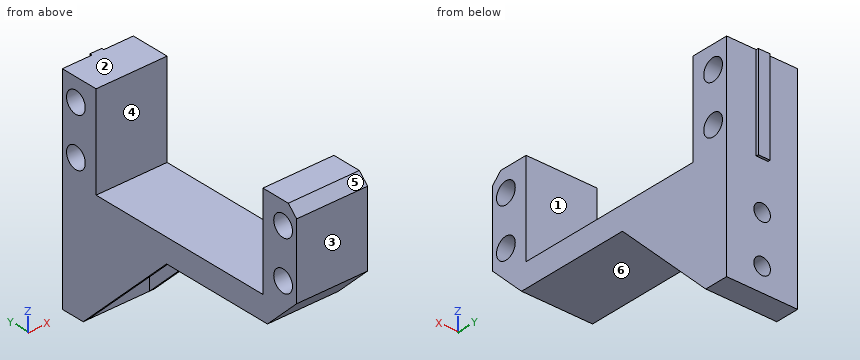
```python
from build123d import *

# Parameters (mm, degrees)
SKETCH019_R             = 2.25
PAD011_DEPTH            = 15
SKETCH020_W             = 20
SKETCH020_H             = 13
POCKET005_DEPTH         = 20
CHAMFER_SIZE            = 19.99
SKETCH021_R             = 1.75
POCKET006_DEPTH         = 5
SKETCH022_W             = 19.8
SKETCH022_H             = 2.5
PAD012_DEPTH            = 0.5
CHAMFER001_SIZE         = 7
CHAMFER002_SIZE         = 2
BODY003_PLACEMENT_ANGLE = 180


with BuildPart() as part:
    # Sketch019 → Pad011 (new body)
    with BuildSketch(Plane.YZ):
        Polygon((-20.02, -9.9), (-28.12, -9.9), (-28.12, 14.9), (3.12, 14.9), (3.12, 34.9), (23.12, 34.9), (28.12, 34.9), (28.12, -9.9), (20.02, -9.9), (20.02, 9.9), (-20.02, 9.9), align=None)
        with Locations((-24.87, -5.15)):
            Circle(SKETCH019_R, mode=Mode.SUBTRACT)
        with Locations((-24.87, 5.15)):
            Circle(SKETCH019_R, mode=Mode.SUBTRACT)
        with Locations((24.87, -5.15)):
            Circle(SKETCH019_R, mode=Mode.SUBTRACT)
        with Locations((24.87, 5.15)):
            Circle(SKETCH019_R, mode=Mode.SUBTRACT)
    extrude(amount=PAD011_DEPTH)

    # Sketch020 (on Face5 of Pad011) → Pocket005 (cut)
    with BuildSketch(Plane(origin=(0, 3.12, 0), x_dir=(0, 0, -1), z_dir=(0, -1, 0))):
        with Locations((-24.9, 7.5)):
            Rectangle(SKETCH020_W, SKETCH020_H)
    extrude(amount=-POCKET005_DEPTH, mode=Mode.SUBTRACT)

    # Chamfer
    chamfer_edges = [part.edges().sort_by_distance(p)[0] for p in [
        (14.5, 3.12, 34.9),
        (0.5, 3.12, 34.9),
    ]]
    chamfer(chamfer_edges, length=CHAMFER_SIZE)

    # Sketch021 (on Face9 of Chamfer) → Pocket006 (cut)
    with BuildSketch(Plane.ZX.offset(28.12)):
        with Locations((19.9, 7.5)):
            Circle(SKETCH021_R)
        with Locations((29.9, 7.5)):
            Circle(SKETCH021_R)
    extrude(amount=-POCKET006_DEPTH, mode=Mode.SUBTRACT)

    # Sketch022 (on Face9 of Pocket006) → Pad012 (join)
    with BuildSketch(Plane.ZX.offset(28.12)):
        with Locations((0, 7.5)):
            Rectangle(SKETCH022_W, SKETCH022_H)
    extrude(amount=PAD012_DEPTH)

    # Chamfer001
    chamfer001_edges = [part.edges().sort_by_distance(p)[0] for p in [
        (7.5, -28.12, 14.9),
    ]]
    chamfer(chamfer001_edges, length=CHAMFER001_SIZE)

    # Chamfer002
    chamfer002_edges = [part.edges().sort_by_distance(p)[0] for p in [
        (7.5, -28.12, -9.9),
    ]]
    chamfer(chamfer002_edges, length=CHAMFER002_SIZE)


with BuildPart() as part_1:
    # Body003 placement: moved
    add(part.part.moved(Location((6.82, 12.82, -27.56))).rotate(Axis((6.82, 12.82, -27.56), (0, 1, 0)), BODY003_PLACEMENT_ANGLE))


solid = part_1.part
```
CAD build for the part. Positions are in the model's coordinates, mm. Face numbers are marked on the shaded views. A direction names the side the tool comes from. Round coordinates to 2 decimals unless told otherwise and drop trailing zeros. Order: outer loops, then holes, each group sorted by start corner. A loop starts at its lowest first (then second) coordinate and runs counter-clockwise, first axis right, second up. Notation, with made-up numbers: (-26, 18) - (-2, 18) arc R33 cw to (-2, 46) - close; hole circle Ø3 at (-27, -11.75). An arc over 180 degrees is marked (long way). Answer in a Markdown table with one row per item. Add a question column.
(1) Band-saw the part on B-B on x = -0.68. List the corners of the cut face in (y, z), and give its area (3 significant figures).
(2) Probe L1, parallel to Y at x = 0.75, z = -32.71; L2, parallel to Y at x = 0, z = -32.71; L3, parallel to Z at x = -1.5, y = -12.05. List the from-to ranges inside material, lowest first. Write a range as [from, to].
(3) Mould opens along Y. For the marked faces 1, 2 and 3 say: +Y half, -Y half, draft (parallel to the pull), parting line (faces both ways), or undercut.
(4) 3-axis set-ups, long thin cutter, end or side, ignore diameter. For the marked faces 4, 5 and 6: which of +Z, -Z, +X, -X, +Y, -Y reach the whole face in a straight line?
(5) Band-saw the part on D-D on z = -47.46. List the corners of the cut face in (x, y).
(6) Band-saw the part on C-C on z = -32.71. List the corners of the cut face in (x, y), and give its area (3 significant figures).
(7) Band-saw the part on A-A on y = 37.69. List the corners of the cut face in (x, z), and give its area (3 significant figures).
(8) Drop flat-ended pins along their axis: pin 1 Ø6.5 at (x, z) = (-1, -57) entering from -Y; pin 2 Ø5 at (x, y) = (4, 33.5) entering from -Z; pin 3 Ø2 at (x, y) = (-4, 22) entering from +Z; pin 4 Ø2.5 at (y, z) = (37.69, -22.41) entering from +X. Give the stop position or say it passes through.
Data:
| question | item | result |
|---|---|---|
| 1 | outline | (-15.3, -35.46) - (-8.3, -42.46) - (35.94, -42.46) - (35.94, -45.71) - (40.94, -45.71) - (40.94, -37.46) - (41.44, -37.46) - (41.44, -17.66) - (32.84, -17.66) - (32.84, -37.46) - (-7.2, -37.46) - (-7.2, -17.66) - (-13.3, -17.66) - (-15.3, -19.66) - close; (35.94, -62.46) - (40.94, -62.46) - (40.94, -59.21) - (35.94, -59.21) - close; (35.94, -55.71) - (40.94, -55.71) - (40.94, -49.21) - (35.94, -49.21) - close; hole circle Ø4.5 at (-12.05, -32.71); hole circle Ø4.5 at (-12.05, -22.41); hole circle Ø4.5 at (37.69, -32.71); hole circle Ø4.5 at (37.69, -22.41) |
| 1 | area | 587 mm^2 |
| 2 | L1 | y = [-15.3, -14.3], [-9.8, -7.2], [32.84, 35.44], [39.94, 40.94] |
| 2 | L2 | y = [-15.3, -14.3], [-9.8, -7.2], [32.84, 35.44], [39.94, 41.44] |
| 2 | L3 | z = [-38.71, -34.96], [-30.46, -24.66], [-20.16, -17.66] |
| 3 | face 1 | undercut |
| 3 | face 2 | draft |
| 3 | face 3 | -Y half |
| 4 | face 4 | +Z, +X, -X |
| 4 | face 5 | +Z, +X, -X, -Y |
| 4 | face 6 | -Z, -Y |
| 5 | outline | (-8.18, 20.93) - (-7.18, 20.93) - (-7.18, 35.94) - (-2.43, 35.94) - (-2.43, 40.94) - (-8.18, 40.94) - close; (1.07, 35.94) - (5.82, 35.94) - (5.82, 20.93) - (6.82, 20.93) - (6.82, 40.94) - (1.07, 40.94) - close |
| 6 | outline | (-8.18, -15.3) - (6.82, -15.3) - (6.82, -14.3) - (-8.18, -14.3) - close; (-8.18, -9.8) - (6.82, -9.8) - (6.82, -7.2) - (-8.18, -7.2) - close; (-8.18, 32.84) - (6.82, 32.84) - (6.82, 35.44) - (-8.18, 35.44) - close; (-8.18, 39.94) - (6.82, 39.94) - (6.82, 40.94) - (0.57, 40.94) - (0.57, 41.44) - (-1.93, 41.44) - (-1.93, 40.94) - (-8.18, 40.94) - close |
| 6 | area | 109 mm^2 |
| 7 | outline | (-8.18, -62.46) - (6.82, -62.46) - (6.82, -34.96) - (-8.18, -34.96) - close; (-8.18, -30.46) - (6.82, -30.46) - (6.82, -24.66) - (-8.18, -24.66) - close; (-8.18, -20.16) - (6.82, -20.16) - (6.82, -17.66) - (-8.18, -17.66) - close; hole circle Ø3.5 at (-0.68, -57.46); hole circle Ø3.5 at (-0.68, -47.46) |
| 7 | area | 518 mm^2 |
| 8 | pin 1 | stops at y = 35.94 |
| 8 | pin 2 | stops at z = -62.46 |
| 8 | pin 3 | stops at z = -37.46 |
| 8 | pin 4 | passes through |
